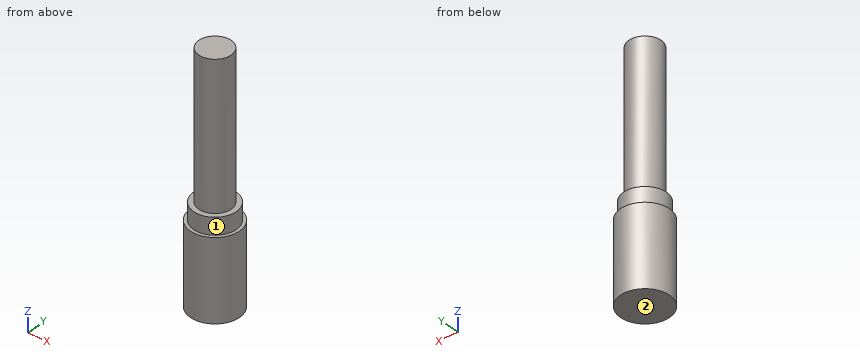
```python
from build123d import *

# Parameters (mm, degrees)
F0_R     = 15.31
F1_DEPTH = 150.27
F2_R     = 15.31
F2_R_2   = 13.33
F3_DEPTH = 100.05
F4_R     = 13.33
F4_R_2   = 10.09
F5_DEPTH = 89.580001


with BuildPart() as f1:
    # F0 (on Top) → F1 (new body)
    with BuildSketch(Plane.XY):
        Circle(F0_R)
    extrude(amount=F1_DEPTH)

    # F2 (on face) → F3 (cut)
    with BuildSketch(Plane.XY.offset(150.27)):
        Circle(F2_R)
        Circle(F2_R_2, mode=Mode.SUBTRACT)
    extrude(amount=-F3_DEPTH, mode=Mode.SUBTRACT)

    # F4 (on face) → F5 (cut)
    with BuildSketch(Plane.XY.offset(150.27)):
        Circle(F4_R)
        Circle(F4_R_2, mode=Mode.SUBTRACT)
    extrude(amount=-F5_DEPTH, mode=Mode.SUBTRACT)


solid = f1.part
```
CAD build for the part. Positions are in the model's coordinates, mm. Face numbers are marked on the shaded views. A direction names the side the tool comes from. Coordinates: 2 decimals unless noted, no trailing zeros. Order: outer loops, then holes, each group sorted by start corner. A loop starts at its lowest first (then second) coordinate and runs counter-clockwise, first axis right, second up.
(1) Drill centre lines: L1, parallel to Z at x = 13.5, y = -4; L2, parallel to Z at x = -13, y = -2.5; L3, parallel to Y at x = 0.5, z = 143.5. Where is each one in solid material? Low to high.
Solution:
L1: z = 0 to 50.22
L2: z = 0 to 60.69
L3: y = -10.08 to 10.08
(2) Saw through at D-D, the plane x = -2. Write the cut outline in (y, z), and give its area (3 significant figures).
Solution:
outline: (-15.18, 0) - (15.18, 0) - (15.18, 50.22) - (13.18, 50.22) - (13.18, 60.69) - (9.89, 60.69) - (9.89, 150.27) - (-9.89, 150.27) - (-9.89, 60.69) - (-13.18, 60.69) - (-13.18, 50.22) - (-15.18, 50.22) - close
area: 3,570 mm2
(3) Saw through at A-A, the plane y = 0. Write the cut outline in (x, z).
Solution:
outline: (-15.31, 0) - (15.31, 0) - (15.31, 50.22) - (13.33, 50.22) - (13.33, 60.69) - (10.09, 60.69) - (10.09, 150.27) - (-10.09, 150.27) - (-10.09, 60.69) - (-13.33, 60.69) - (-13.33, 50.22) - (-15.31, 50.22) - close
(4) Saw through at C-C, the plane z = 58. Write the cut outline in (x, y), and give its area (3 significant figures).
Solution:
outline: circle Ø26.66 at (0, 0)
area: 558 mm2
(5) Pin check, flat tips, straight feed: pin 1 Ø4 at (x, z) = (-6, 20) entering from +Y; pin 2 Ø10 at (y, z) = (0, 75.5) entering from +X; pin 3 Ø4 at (x, z) = (7.5, 74.5) entering from -Y. Stop position of each tip, or through.
Solution:
pin 1: stops at y = 14.78
pin 2: stops at x = 10.09
pin 3: stops at y = -8.46
(6) Which spindle directions (+Z, -Z, +X, -X, +Y, -Y) get a long thin tool onto all of the face, cutting with end or side? Do the marked faces 1 and 2. Say none if no direction does.
Solution:
face 1: +Z
face 2: -Z, +X, -X, +Y, -Y
(7) Saw through at B-B, the plane x = -11.5. Write the cut outline in (y, z).
Solution:
outline: (-10.11, 0) - (10.11, 0) - (10.11, 50.22) - (6.74, 50.22) - (6.74, 60.69) - (-6.74, 60.69) - (-6.74, 50.22) - (-10.11, 50.22) - close
